from build123d import *

# Parameters (mm, degrees)
SKETCH4_W           = 3.872983346
SKETCH4_H           = 1
BOSS_EXTRUDE1_DEPTH = 8


with BuildPart() as part:
    # Sketch2 → Revolve1 (revolve)
    with BuildSketch(Plane.XY, mode=Mode.PRIVATE) as revolve1_sk:
        Polygon((0, 0), (0, 50), (0, 53), (5, 53), (5, 50), (2.5, 50), (2.5, 5), (2, 5), (2, 0), align=None)
    revolve(revolve1_sk.sketch.rotate(Axis((0, 0, 0), (0, 1, 0)), 90), axis=Axis((0, 0, 0), (0, 1, 0)))

    # Sketch4 → Boss-Extrude1 (add)
    with BuildSketch(Plane.XZ):
        Rectangle(SKETCH4_W, SKETCH4_H)
    extrude(amount=BOSS_EXTRUDE1_DEPTH)


solid = part.part
Design review of the part built by this model. Coordinates are the model's own, in mm. A direction names the side the tool comes from. Coordinates: 2 decimals unless noted, no trailing zeros. Order: outer loops, then holes, each group sorted by start corner. A loop starts at its lowest first (then second) coordinate and runs counter-clockwise, first axis right, second up.
Item 1: Take a section at B-B, the plane y = -3. Write out the cut boundary in (x, z).
Item 2: For pin 1 Ø1.6 at (x, z) = (-0.5, -1) entering from -Y; pin 2 Ø1.1 at (y, z) = (-5, 0) entering from +X; pin 3 Ø1.2 at (x, y) = (-1, -4.5) entering from +Z; pin 4 Ø6 at (y, z) = (-1, 2.5) entering from -X, all flat-tipped, find the tip position at first contact; note any pin that passes through.
Item 3: Take a section at C-C, the plane z = 3.75. Write out the cut boundary in (x, y).
Item 4: For faces 1 (the cylindrical face through (-0.1, 27.2, 2.5)), 2 (the flat face through (1.936, -4, 0)), 3 (the flat face through (-1.936, -4, 0)), 4 (the flat face through (0, -4, 0.5)), 5 (the flat face through (0, -4, -0.5)), list the 3-axis set-ups (+Z, -Z, +X, -X, +Y, -Y) from which the entire face can be reached by the end or side of a thin tool; tool diameter is ignored.
Item 5: Take a section at D-D, the plane y = 18. Write out the cut boundary in (x, z).
Item 6: For line 1 (Y direction, x = 3.75, z = 0); line 2 (Z direction, x = 1.5, y = 30); line 3 (Y direction, x = 2.25, z = -1), list the stretches that pass through material, from the lowest coordinate up.
Item 7: Take a section at A-A, the plane x = 0. Write out the cut boundary in (y, z).
The answers:
1. outline: (-1.94, -0.5) - (1.94, -0.5) - (1.94, 0.5) - (-1.94, 0.5) - close
2. pin 1: stops at y = -8
2. pin 2: stops at x = 1.94
2. pin 3: stops at z = 0.5
2. pin 4: stops at x = -2
3. outline: (-3.31, 50) - (3.31, 50) - (3.31, 53) - (-3.31, 53) - close
4. face 1: -Y
4. face 2: +Z, -Z, +X, -Y
4. face 3: +Z, -Z, -X, -Y
4. face 4: +Z, +X, -X, -Y
4. face 5: -Z, +X, -X, -Y
5. outline: circle Ø5 at (0, 0)
6. line 1: y = 50 to 53
6. line 2: z = -2 to 2
6. line 3: y = 5 to 53
7. outline: (-8, -0.5) - (0, -0.5) - (0, -2) - (5, -2) - (5, -2.5) - (50, -2.5) - (50, -5) - (53, -5) - (53, 5) - (50, 5) - (50, 2.5) - (5, 2.5) - (5, 2) - (0, 2) - (0, 0.5) - (-8, 0.5) - close
